For this review, use the dimensioned drawing (mm, ordinates from the lowest corner) and the shaded views. A direction names the side the tool comes from. Round coordinates to 2 decimals unless told otherwise and drop trailing zeros. Order: outer loops, then holes, each group sorted by start corner. A loop starts at its lowest first (then second) coordinate and runs counter-clockwise, first axis right, second up. Notation, with made-up numbers: M 7,-2 L 43,-2 A6 cw 43,6 Z; hole C -28,60.25 d3. An arc over 180 degrees is marked long. Use a Markdown table: item, result. Add a question column.
1. Consider section C-C on z = 7.25. State the section outline as (x, y) points.
2. To check wall thickness, follow probe 1 along Y at (x, z) = (35, 8.25); probe 2 along Y at (x, z) = (19, 8.25); probe 3 along X at (y, z) = (6.5, 6.45). State the ranges of each line that lie inside material, in increasing order.
3. The part is to be moulded in two halves that separate along Y. For the marked faces 3, 4 and 5, say which applies: +Y half, -Y half, draft (parallel to the pull), parting line (faces both ways), or undercut.
4. Consider section B-B on x = 19. State the section outline as (y, z) points.
5. Consider section A-A on y = 6.5. State the section outline as (x, z) points, then the cut area to 3 significant figures.
6. For the marked faces 1 and 2, list the 3-axis set-ups (+Z, -Z, +X, -X, +Y, -Y) from which the entire face can be reached by the end or side of a thin tool; tool diameter is ignored.
7. Consider section D-D on y = 21.5. State the section outline as (x, z) points, then the cut area to 3 significant figures.
8. Insertion check: P1, Ø4, axis at y = 17.5, z = 6.5, coming from the +X side (1 decimal); P2, Ø7, axis at x = 19, y = 31.5, coming from the +Z side; P3, Ø6, axis at y = 6.5, z = 5, coming from the -X side. Each pin has a flat end and moves straight along its axis. Give the tip position at first contact, or say it passes through.
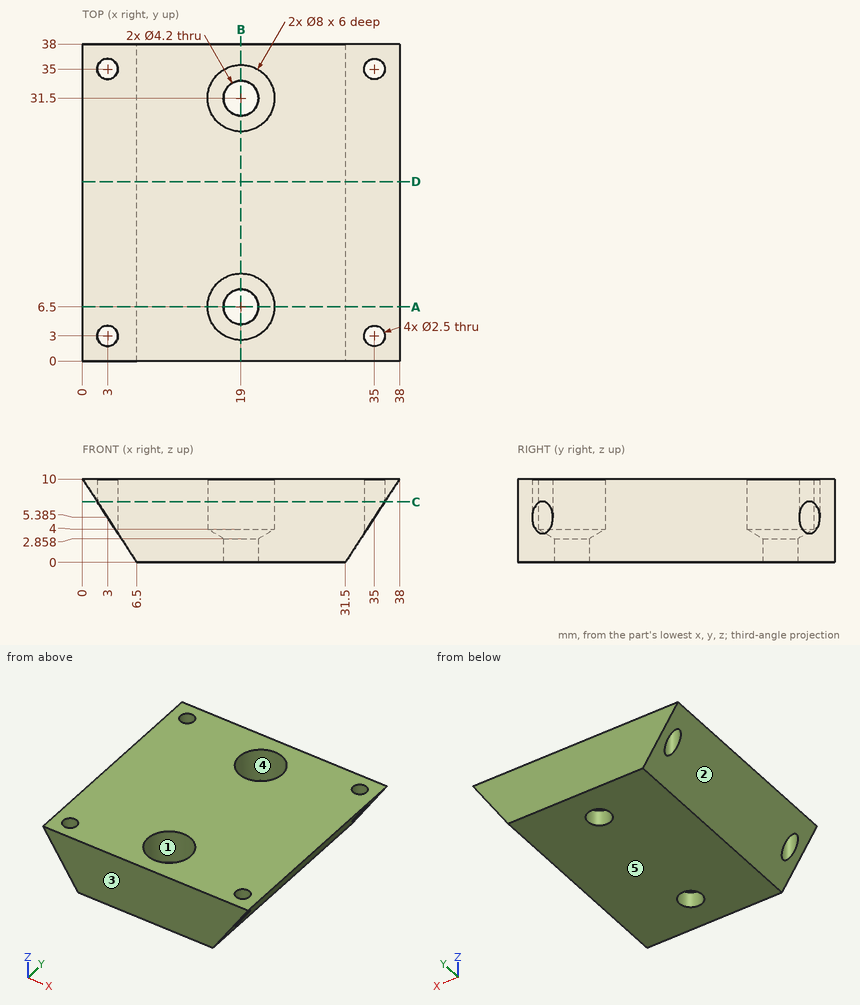
Answer block:
| question | item | result |
|---|---|---|
| 1 | outline | M 1.79,0 L 36.21,0 L 36.21,2.7 A1.25 cw long 36.21,3.3 L 36.21,34.7 A1.25 cw long 36.21,35.3 L 36.21,38 L 1.79,38 L 1.79,35.3 A1.25 cw long 1.79,34.7 L 1.79,3.3 A1.25 cw long 1.79,2.7 Z; hole C 19,6.5 d8; hole C 19,31.5 d8 |
| 2 | probe 1 | 0 to 1.75, 4.25 to 33.75, 36.25 to 38 |
| 2 | probe 2 | 0 to 2.5, 10.5 to 27.5, 35.5 to 38 |
| 2 | probe 3 | 2.31 to 15, 23 to 35.69 |
| 3 | face 3 | -Y half |
| 3 | face 4 | undercut |
| 3 | face 5 | draft |
| 4 | outline | M 0,0 L 4.4,0 L 4.4,2.86 L 2.5,4 L 2.5,10 L 0,10 Z; M 8.6,0 L 29.4,0 L 29.4,2.86 L 27.5,4 L 27.5,10 L 10.5,10 L 10.5,4 L 8.6,2.86 Z; M 33.6,0 L 38,0 L 38,10 L 35.5,10 L 35.5,4 L 33.6,2.86 Z |
| 5 | outline | M 0,10 L 6.5,0 L 16.9,0 L 16.9,2.86 L 15,4 L 15,10 Z; M 21.1,0 L 31.5,0 L 38,10 L 23,10 L 23,4 L 21.1,2.86 Z |
| 5 | area | 248 mm^2 |
| 6 | face 1 | +Z |
| 6 | face 2 | -Z, -X, +Y, -Y |
| 7 | outline | M 0,10 L 6.5,0 L 31.5,0 L 38,10 Z |
| 7 | area | 315 mm^2 |
| 8 | P1 | x = 37 |
| 8 | P2 | z = 3.7 |
| 8 | P3 | x = 1.3 |
